Read the model definition and answer for the solid it produces. Units are mm, in the model's axes. Coordinates: 2 decimals unless noted, no trailing zeros. Write each loop counter-clockwise with the first axis right and the second up, starting at its lowest first coordinate (ties: lowest second). Pieces come first, ordered by that corner, then holes.
(1) The part is cut by section B-B, the plane x = -32. Determine the outline of the cut face in (y, z).
(2) Given pin 1 (1.5 mm diameter, centred on y = -10, z = 2, fed in from +X); pin 2 (1 mm diameter, centred on x = 1, z = 2.5, fed in from -Y), each flat-ended and moving along its own axis, determine where each tip first touches the part or whether it passes through.
(3) The part is cut by section D-D, the plane z = 0.65. Determine the outline of the cut face in (x, y), and give its area (3 significant figures).
(4) Straight lines are drawn through the part: line 1 along Y through (x, z) = (7, 1.05); line 2 along Y through (x, z) = (13.5, 1.35); line 3 along X through (y, z) = (-12, 2.5). For each, find the intervals that lie inside material, in ascending order.
(5) The part is cut by section A-A, the plane y = -13.5. Determine the outline of the cut face in (x, z).
(6) The part is cut by section C-C, the plane y = -5.5. Determine the outline of the cut face in (x, z), and give its area (3 significant figures).
```python
from build123d import *

# Parameters (mm, degrees)
F0_R     = 11
F1_DEPTH = 3


with BuildPart() as f1:
    # F0 (on Top) → F1 (new body)
    with BuildSketch(Plane.XY):
        with BuildLine():
            ThreePointArc((0, -11), (9.526279, -5.5), (9.526279, 5.5))
            ThreePointArc((9.526279, 5.5), (5.5, 9.526279), (0, 11))
            ThreePointArc((0, 11), (-5.5, 9.526279), (-9.526279, 5.5))
            ThreePointArc((-9.526279, 5.5), (-9.526279, -5.5), (0, -11))
        make_face()
        with BuildLine():
            ThreePointArc((11, 27), (-7.778175, 34.778175), (0, 16))
            ThreePointArc((0, 16), (7.778175, 19.221825), (11, 27))
        make_face()
        with BuildLine():
            ThreePointArc((14.960517, -1.087624), (14.620192, 3.354102), (12.990381, 7.5))
            ThreePointArc((12.990381, 7.5), (10.214833, 10.984406), (6.538348, 13.5))
            ThreePointArc((6.538348, 13.5), (0, 42), (-6.538348, 13.5))
            ThreePointArc((-6.538348, 13.5), (-10.214833, 10.984406), (-12.990381, 7.5))
            ThreePointArc((-12.990381, 7.5), (-14.620192, 3.354102), (-14.960517, -1.087624))
            ThreePointArc((-14.960517, -1.087624), (-36.373067, -21), (-8.422169, -12.412376))
            ThreePointArc((-8.422169, -12.412376), (-4.405358, -14.338508), (0, -15))
            ThreePointArc((0, -15), (4.405358, -14.338508), (8.422169, -12.412376))
            ThreePointArc((8.422169, -12.412376), (36.373067, -21), (14.960517, -1.087624))
        make_face()
        with Locations((-23.382686, -13.5)):
            Circle(F0_R, mode=Mode.SUBTRACT)
        with Locations((23.382686, -13.5)):
            Circle(F0_R, mode=Mode.SUBTRACT)
        with BuildLine():
            ThreePointArc((0, 11), (5.5, 9.526279), (9.526279, 5.5))
            ThreePointArc((9.526279, 5.5), (9.526279, -5.5), (0, -11))
            ThreePointArc((0, -11), (-9.526279, -5.5), (-9.526279, 5.5))
            ThreePointArc((-9.526279, 5.5), (-5.5, 9.526279), (0, 11))
        make_face(mode=Mode.SUBTRACT)
        with BuildLine():
            ThreePointArc((11, 27), (7.778175, 19.221825), (0, 16))
            ThreePointArc((0, 16), (-7.778175, 34.778175), (11, 27))
        make_face(mode=Mode.SUBTRACT)
    extrude(amount=F1_DEPTH)


solid = f1.part
```
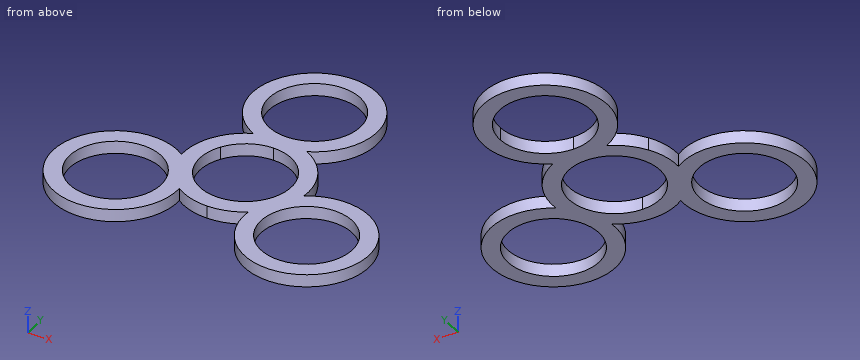
Computed:
1. outline: (-25.78, 0) - (-20.34, 0) - (-20.34, 3) - (-25.78, 3) - close; (-6.66, 0) - (-1.22, 0) - (-1.22, 3) - (-6.66, 3) - close
2. pin 1: stops at x = 38.13
2. pin 2: stops at y = -14.99
3. outline: (-14.96, -1.09) arc R15 ccw (long way) to (-8.42, -12.41) arc R15 ccw to (0, -15) arc R15 ccw to (8.42, -12.41) arc R15 ccw (long way) to (14.96, -1.09) arc R15 ccw to (12.99, 7.5) arc R15 ccw to (6.54, 13.5) arc R15 ccw (long way) to (-6.54, 13.5) arc R15 ccw to (-12.99, 7.5) arc R15 ccw to start; hole circle Ø22 at (-23.38, -13.5); hole (-9.53, 5.5) arc R11 ccw (long way) to (9.53, 5.5) arc R11 ccw to (0, 11) arc R11 ccw to start; hole (0, 16) arc R11 ccw to (11, 27) arc R11 ccw (long way) to start; hole circle Ø22 at (23.38, -13.5)
3. area: 1,230 mm2
4. line 1: y = -13.27 to -8.49, 8.49 to 13.27, 13.73 to 18.51, 35.49 to 40.27
4. line 2: y = -24.78 to -18.33, -8.67 to 6.54, 20.46 to 33.54
4. line 3: x = -38.31 to -34.28, -12.49 to 12.49, 34.28 to 38.31
5. outline: (-38.38, 0) - (-34.38, 0) - (-34.38, 3) - (-38.38, 3) - close; (-12.38, 0) - (-8.38, 0) - (-8.38, 3) - (-12.38, 3) - close; (-6.54, 0) - (6.54, 0) - (6.54, 3) - (-6.54, 3) - close; (8.38, 0) - (12.38, 0) - (12.38, 3) - (8.38, 3) - close; (34.38, 0) - (38.38, 0) - (38.38, 3) - (34.38, 3) - close
6. outline: (-36.07, 0) - (-30.93, 0) - (-30.93, 3) - (-36.07, 3) - close; (-15.83, 0) - (-9.53, 0) - (-9.53, 3) - (-15.83, 3) - close; (9.53, 0) - (15.83, 0) - (15.83, 3) - (9.53, 3) - close; (30.93, 0) - (36.07, 0) - (36.07, 3) - (30.93, 3) - close
6. area: 68.7 mm2
